Design review of the part built by this model. Coordinates are the model's own, in mm. A direction names the side the tool comes from. Round coordinates to 2 decimals unless told otherwise and drop trailing zeros. Order: outer loops, then holes, each group sorted by start corner. A loop starts at its lowest first (then second) coordinate and runs counter-clockwise, first axis right, second up. Notation, with made-up numbers: M 28.25,8 L 85.25,8 A12 ccw 85.25,23 Z; hole C -10.5,-14 d7. An arc over 180 degrees is marked long. Write item = value, one per line. Start each with the question number.
```python
from build123d import *

# Parameters (mm, degrees)
F1_DEPTH = 25.4
F0_R     = 1.27
F0_R_2   = 2.54
F2_DEPTH = 15.24
F3_DEPTH = 10.16
F4_DEPTH = 12.7


with BuildPart() as f1:
    # F0 (on Top) → F1 (new body)
    with BuildSketch(Plane.XY):
        Polygon((-9.525, -91.6940000873), (9.525, -91.6940000873), (9.525, -4.0542031638), (-9.525, -4.0542031638), (-9.525, -6.5866475925), (-9.525, -7.8647015616), align=None)
        Polygon((5.7174111716, -90.4213413596), (-5.7059712708, -90.4213413596), (0.0057199504, -56.1548753595), align=None, mode=Mode.SUBTRACT)
        Polygon((-6.9876490161, -9.1256853193), (-0.2122831974, -49.7735133395), (-6.7739198121, -89.1391038895), align=None, mode=Mode.SUBTRACT)
        Polygon((0.210035916, -49.7735133395), (6.9854017347, -9.1256853193), (6.7716725307, -89.1391038895), align=None, mode=Mode.SUBTRACT)
        Polygon((-5.7059712708, -7.8647015616), (5.7174111716, -7.8647015616), (0.0057199504, -42.1311675618), align=None, mode=Mode.SUBTRACT)
    extrude(amount=-F1_DEPTH)

    # F0 (on Top) → F2 (join)
    with BuildSketch(Plane.XY):
        with BuildLine():
            Line((-9.525, -4.0542031638), (9.525, -4.0542031638))
            Line((9.525, -4.0542031638), (9.525, 21.3359999127))
            Line((9.525, 21.3359999127), (14.2927857936, 29.5818378705))
            ThreePointArc((14.2927857936, 29.5818378705), (0, 54.3559999127), (-14.2927857936, 29.5818378705))
            Line((-14.2927857936, 29.5818378705), (-9.525, 21.3359999127))
            Line((-9.525, 21.3359999127), (-9.525, 2.7279353235))
            Line((-9.525, 2.7279353235), (-9.525, -4.0542031638))
        make_face()
        with Locations((0, 24.5959999127)):
            Circle(F0_R, mode=Mode.SUBTRACT)
        with Locations((-13.25, 37.8459999127)):
            Circle(F0_R, mode=Mode.SUBTRACT)
        with Locations((0, 37.8459999127)):
            Circle(F0_R_2, mode=Mode.SUBTRACT)
        with Locations((0, 51.0959999127)):
            Circle(F0_R, mode=Mode.SUBTRACT)
        with Locations((13.25, 37.8459999127)):
            Circle(F0_R, mode=Mode.SUBTRACT)
    extrude(amount=-F2_DEPTH)

    # F0 (on Top) → F3 (cut)
    with BuildSketch(Plane.XY):
        with BuildLine():
            Line((-9.525, -4.0542031638), (9.525, -4.0542031638))
            Line((9.525, -4.0542031638), (9.525, 21.3359999127))
            Line((9.525, 21.3359999127), (14.2927857936, 29.5818378705))
            ThreePointArc((14.2927857936, 29.5818378705), (0, 54.3559999127), (-14.2927857936, 29.5818378705))
            Line((-14.2927857936, 29.5818378705), (-9.525, 21.3359999127))
            Line((-9.525, 21.3359999127), (-9.525, 2.7279353235))
            Line((-9.525, 2.7279353235), (-9.525, -4.0542031638))
        make_face()
        with Locations((0, 24.5959999127)):
            Circle(F0_R, mode=Mode.SUBTRACT)
        with Locations((-13.25, 37.8459999127)):
            Circle(F0_R, mode=Mode.SUBTRACT)
        with Locations((0, 37.8459999127)):
            Circle(F0_R_2, mode=Mode.SUBTRACT)
        with Locations((0, 51.0959999127)):
            Circle(F0_R, mode=Mode.SUBTRACT)
        with Locations((13.25, 37.8459999127)):
            Circle(F0_R, mode=Mode.SUBTRACT)
    extrude(amount=-F3_DEPTH, mode=Mode.SUBTRACT)

    # F0 (on Top) → F4 (join)
    with BuildSketch(Plane.XY):
        Polygon((44.5479988722, -127.9869989595), (9.525, -92.9640000873), (9.525, -91.6940000873), (-9.525, -91.6940000873), (-9.525, -92.9640000873), (1.1633583069, -102.417688386), (2.114645682, -103.2590874174), (45.4460244843, -141.5850245716), (46.7160244843, -141.5850245716), (81.0060244843, -141.5850245716), (83.5460244843, -141.5850245716), (83.5460244843, -139.0450245716), (83.5460244843, -131.4250245716), (83.5460244843, -128.8850245716), (45.4460244843, -128.8850245716), align=None)
        Polygon((26.5501800765, -113.5745529767), (42.7553124657, -129.7796853659), (39.5531307355, -132.9818670961), (22.6265746152, -118.0105889131), align=None, mode=Mode.SUBTRACT)
        Polygon((3.7974437448, -101.3565126673), (8.741913116, -95.7662860163), (24.7524432855, -111.7768161858), (20.7257820574, -116.3293671719), align=None, mode=Mode.SUBTRACT)
        Polygon((46.7160244843, -132.6950245716), (58.1460244843, -135.2350245716), (46.7160244843, -137.7750245716), align=None, mode=Mode.SUBTRACT)
        Polygon((79.7360244843, -139.0450245716), (47.9860244843, -139.0450245716), (63.8610244843, -135.5172467938), align=None, mode=Mode.SUBTRACT)
        Polygon((47.9860244843, -131.4250245716), (79.7360244843, -131.4250245716), (63.8610244843, -134.9528023494), align=None, mode=Mode.SUBTRACT)
        Polygon((81.0060244843, -132.6950245716), (81.0060244843, -137.7750245716), (69.5760244843, -135.2350245716), align=None, mode=Mode.SUBTRACT)
    extrude(amount=-F4_DEPTH)


solid = f1.part
```
(1) Insertion check: pin 1 (8 mm diameter, centred on x = -0.5, z = -4, fed in from +Y); pin 2 (12 mm diameter, centred on y = 21, z = -3.5, fed in from -X); pin 3 (6 mm diameter, centred on x = 4.5, z = -15, fed in from -Y); pin 4 (2.5 mm diameter, centred on y = -136.5, z = -6.5, fed in from -X). Each pin has a flat end and moves straight along its axis. Give the tip position at first contact, or say it passes through.
(2) For faces 1 (the face through (9, -72, 0)), 2 (the face through (9.525, -49, -13)), 3 (the face through (0, -47, -25.4)), 4 (the face through (22.77, -114.02, -6.26)), 5 (the face through (0, -4.054, -20)), list the 3-axis set-ups (+Z, -Z, +X, -X, +Y, -Y) from which the entire face can be reached by the end or side of a thin tool; tool diameter is ignored.
(3) Consider section B-B, the plane y = -18. Write out the cut boundary in (x, z) (3 decimals).
(4) Draft analysis for pull direction Y (two halves, no side actions). For faces 6 (the face through (0, -91.694, -19)), 7 (the face through (31.21, -125.6, -6.26)), 8 (the face through (0, -4.054, -5)), state which applies: pulls with the +Y half, pulls with the -Y half, needs draft (parallel to the pull), parting line crosses it, or undercut.
(5) For line 1 along X through (y, z) = (-84.5, -19.75) (3 decimals); line 2 along Y through (x, z) = (13.25, -11.5); line 3 along X through (y, z) = (-78.5, -12.5) (3 decimals), list the stretches that pass through material, from the lowest coordinate up. Write a range as [from, to].
(6) Consider section C-C, the plane z = -3.5. State how many separate pieces and enclosed holes the cut face has, then the cut area to 3 significant figures.
(7) Consider section A-A, the plane z = -23.5. Write out the cut boundary in (x, y) (3 decimals), then the cut area to 3 significant figures.
Completed:
q1.pin_1 = -4.05
q1.pin_2 = through
q1.pin_3 = -107.07
q1.pin_4 = 38.28
q2.face_1 = +Z, +X, -X, +Y, -Y
q2.face_2 = +Z, -Z, +X
q2.face_3 = -Z, +X, -X, +Y, -Y
q2.face_4 = +Z, -Z
q2.face_5 = -Z, +X, -X, +Y
q3.outline = M -9.525,-25.4 L -6.964,-25.4 L -6.964,0 L -9.525,0 Z; M -5.508,-25.4 L -4.017,-25.4 L -4.017,0 L -5.508,0 Z; M 4.028,-25.4 L 5.506,-25.4 L 5.506,0 L 4.028,0 Z; M 6.962,-25.4 L 9.525,-25.4 L 9.525,0 L 6.962,0 Z
q4.face_6 = pulls with the -Y half
q4.face_7 = undercut
q4.face_8 = pulls with the +Y half
q5.line_1 = [-9.525, -6.786], [-6.001, -4.719], [4.73, 5.998], [6.784, 9.525]
q5.line_2 = [-113.11, -109.72], [-100.27, -96.69], [27.78, 36.58], [39.12, 47.7]
q5.line_3 = [-9.525, -6.802], [-5.001, -3.719], [3.73, 4.998], [6.8, 9.525]
q6.separate_pieces = 1
q6.enclosed_holes = 10
q6.area = 1,500 mm2
q7.outline = M -9.525,-91.694 L 9.525,-91.694 L 9.525,-4.054 L -9.525,-4.054 Z; hole M -6.988,-9.126 L -6.774,-89.139 L -0.212,-49.774 Z; hole M -5.706,-90.421 L 5.717,-90.421 L 0.006,-56.155 Z; hole M -5.706,-7.865 L 0.006,-42.131 L 5.717,-7.865 Z; hole M 0.21,-49.774 L 6.772,-89.139 L 6.985,-9.126 Z
q7.area = 745 mm2
